Geometry check sheet. Reference: the model listing, model coordinates, mm. Face numbers are marked on the shaded views. A direction names the side the tool comes from. Round coordinates to 2 decimals unless told otherwise and drop trailing zeros. Loops run counter-clockwise (first coordinate to the right, second up) from the corner with the lowest first, then second, coordinate; pieces in that order, holes last. Notation, with made-up numbers: (-26.75, -25.75) -> (-0.75, -25.75) arc R33 cw to (-0.75, 6.25) -> close; hole circle Ø4 at (41.25, 62). An arc over 180 degrees is marked (long way). Use one line per item in the form item = value.
from build123d import *

# Parameters (mm, degrees)
SKETCH1_R           = 95.492297116
BOSS_EXTRUDE1_DEPTH = 100
SKETCH3_3_R         = 32.5
TUBE_DEPTH          = 275
SKETCH5_R           = 82.5
TOP_HUB_DEPTH       = 60
BLADES_DEPTH        = 160
FILLET3_R           = 1.5
FILLET5_R           = 6
FILLET6_R           = 6


with BuildPart() as part:
    # Sketch1 → Boss-Extrude1 (new body)
    with BuildSketch(Plane(origin=(0, 0, 0), x_dir=(1, 0, 0), z_dir=(0, 1, 0))):
        with Locations(Location((0, 0, 0), (0, 0, 270))):
            Circle(SKETCH1_R)
    extrude(amount=BOSS_EXTRUDE1_DEPTH)

    # Loft2: read off the stored shape, not the designer's step
    # Loft2: loft between two sections, ruled curve by curve
    loft2_from = [
        Edge.make_bspline([(30.430707277, 125, -11.411487835), (53.253682947, 125, 49.44992672), (-7.607731608, 125, 72.272902389), (-30.430707277, 125, 11.411487835), (-53.253682947, 125, -49.44992672), (7.607731608, 125, -72.272902389), (30.430707277, 125, -11.411487835)], [0, 0, 0, 0, 0.5, 0.5, 0.5, 1, 1, 1, 1], 3, [1, 0.333333333, 0.333333333, 1, 0.333333333, 0.333333333, 1]),
    ]
    loft2_to = [
        Edge.make_bspline([(87.277179809, 100, 38.748841183), (9.779497444, 100, 213.303200802), (-164.774862175, 100, 135.805518436), (-87.277179809, 100, -38.748841183), (-9.779497444, 100, -213.303200802), (164.774862175, 100, -135.805518436), (87.277179809, 100, 38.748841183)], [0, 0, 0, 0, 0.5, 0.5, 0.5, 1, 1, 1, 1], 3, [1, 0.333333333, 0.333333333, 1, 0.333333333, 0.333333333, 1]),
    ]
    loft2 = Solid(Shell([*[Face.make_surface_from_curves(loft2_from[k], loft2_to[k]) for k in range(1)], Face(Wire(loft2_from)), Face(Wire(loft2_to))]))
    add(loft2)

    # Sketch3<3> → tube (add)
    with BuildSketch(Plane(origin=(0, 125, 0), x_dir=(1, 0, 0), z_dir=(0, 1, 0))):
        with Locations(Location((0, 0, 0), (0, 0, 20.556))):
            Circle(SKETCH3_3_R)
    extrude(amount=TUBE_DEPTH)

    # Sketch5 → top_hub (add)
    with BuildSketch(Plane(origin=(0, 400, 0), x_dir=(1, 0, 0), z_dir=(0, 1, 0))):
        with Locations(Location((0, 0, 0), (0, 0, 270))):
            Circle(SKETCH5_R)
    extrude(amount=TOP_HUB_DEPTH)

    # Sketch8 → Blades (add)
    with BuildSketch(Plane(origin=(0, 460, 0), x_dir=(1, 0, 0), z_dir=(0, 1, 0))):
        with BuildLine():
            ThreePointArc((123.296710019, -36.922200146), (95.784801634, -26.321129354), (82.5, 0))
            ThreePointArc((82.5, 0), (91.565639785, 30.041990229), (119.218910164, 44.874509873))
            Line((119.218910164, 44.874509873), (119.616744296, 40.894343042))
            ThreePointArc((119.616744296, 40.894343042), (94.661353954, 27.508898485), (86.480166831, 0.397834132))
            ThreePointArc((86.480166831, 0.397834132), (98.468890257, -23.355380163), (123.296710019, -32.922200146))
            Line((123.296710019, -32.922200146), (123.296710019, -36.922200146))
        make_face()
        with BuildLine():
            ThreePointArc((-119.218910164, 44.874509873), (-91.565639785, 30.041990229), (-82.5, 0))
            ThreePointArc((-82.5, 0), (-95.784801634, -26.321129354), (-123.296710019, -36.922200146))
            Line((-123.296710019, -36.922200146), (-123.296710019, -32.922200146))
            ThreePointArc((-123.296710019, -32.922200146), (-98.468890257, -23.355380163), (-86.480166831, 0.397834132))
            ThreePointArc((-86.480166831, 0.397834132), (-94.661353954, 27.508898485), (-119.616744296, 40.894343042))
            Line((-119.616744296, 40.894343042), (-119.218910164, 44.874509873))
        make_face()
        with BuildLine():
            ThreePointArc((38.088025782, 119.593401567), (25.871262622, 94.036384856), (0, 82.5))
            ThreePointArc((0, 82.5), (-29.727635854, 92.548615238), (-43.642804778, 120.674672115))
            Line((-43.642804778, 120.674672115), (-39.651708344, 120.941410294))
            ThreePointArc((-39.651708344, 120.941410294), (-27.094116876, 95.559358966), (-0.266738179, 86.491096434))
            ThreePointArc((-0.266738179, 86.491096434), (23.080498822, 96.901980328), (34.105382649, 119.965629555))
            Line((34.105382649, 119.965629555), (38.088025782, 119.593401567))
        make_face()
        with BuildLine():
            ThreePointArc((-43.642804778, -120.674672115), (-29.727635854, -92.548615238), (0, -82.5))
            ThreePointArc((0, -82.5), (25.871262622, -94.036384856), (38.088025782, -119.593401567))
            Line((38.088025782, -119.593401567), (34.105382649, -119.965629555))
            ThreePointArc((34.105382649, -119.965629555), (23.080498822, -96.901980328), (-0.266738179, -86.491096434))
            ThreePointArc((-0.266738179, -86.491096434), (-27.094116876, -95.559358966), (-39.651708344, -120.941410294))
            Line((-39.651708344, -120.941410294), (-43.642804778, -120.674672115))
        make_face()
    extrude(amount=-BLADES_DEPTH)

    # Fillet3
    fillet3_edges = [part.edges().sort_by_distance(p)[0] for p in [
        (123.296710019, 380, 36.922200146),
        (119.218910164, 380, -44.874509873),
        (119.616744296, 380, -40.894343042),
        (123.296710019, 380, 32.922200146),
        (-119.218910164, 380, -44.874509873),
        (-123.296710019, 380, 36.922200146),
        (-123.296710019, 380, 32.922200146),
        (-119.616744296, 380, -40.894343042),
        (38.088025782, 380, -119.593401567),
        (-43.642804778, 380, -120.674672115),
        (-39.651708344, 380, -120.941410294),
        (34.105382649, 380, -119.965629555),
        (-43.642804778, 380, 120.674672115),
        (38.088025782, 380, 119.593401567),
        (34.105382649, 380, 119.965629555),
        (-39.651708344, 380, 120.941410294),
    ]]
    fillet(fillet3_edges, radius=FILLET3_R)

    # Fillet5
    fillet5_edges = [part.edges().sort_by_distance(p)[0] for p in [
        (52.050758656, 100, 80.059336319),
        (-30.430707277, 125, 11.411487835),
    ]]
    fillet(fillet5_edges, radius=FILLET5_R)

    # Fillet6
    fillet6_edges = [part.edges().sort_by_distance(p)[0] for p in [
        (-30.430707277, 400, 11.411487835),
    ]]
    fillet(fillet6_edges, radius=FILLET6_R)


solid = part.part
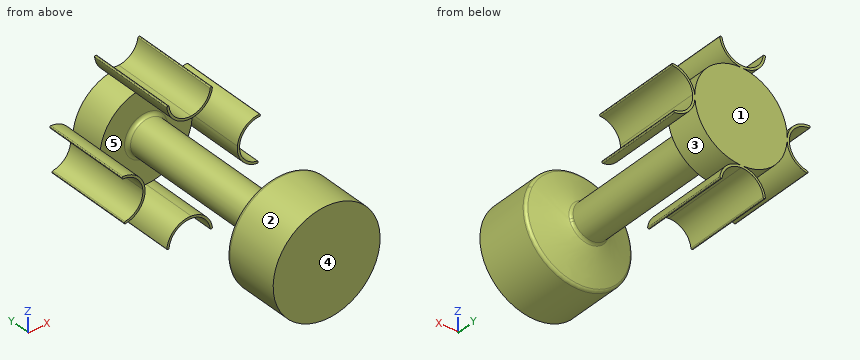
1. Mould release check, pull along Z, two halves, no side actions. Record for the marked faces 1, 2 and 3: released by +Z, released by -Z, zero draft, split by the parting line, or undercut.
Return value:
face_1 = zero draft
face_2 = split by the parting line
face_3 = undercut
2. Gauge pin test, flat ends, axial feed: pin 1 (6 mm diameter, centred on x = -93.5, y = 399.5, fed in from -Z); pin 2 (12 mm diameter, centred on y = 404.5, z = 79, fed in from -X) (3 decimals); pin 3 (2 mm diameter, centred on y = 404.5, z = 70, fed in from +X); pin 4 (5 mm diameter, centred on x = 53.5, z = 9.5, fed in from -Y). Record the tip position at first contact, or that the pin passes through.
Return value:
pin_1 = -35.11
pin_2 = -38.435
pin_3 = 45.22
pin_4 = 0
3. Section check A-A (z = 102.5). Record the boundary of the cut face in (x, y).
Return value:
outline = (-38, 300) -> (-33.26, 300) -> (-33.26, 460) -> (-38, 460) -> close; (27.79, 300) -> (32.53, 300) -> (32.53, 460) -> (27.79, 460) -> close
4. Tool access check on the marked faces 4 and 5. Record the directions out of +Z, -Z, +X, -X, +Y, -Y that give a thin tool (end or side, any length) a straight path to the whole face; none if there is none.
Return value:
face_4 = +Z, -Z, +X, -X, -Y
face_5 = none
5. Section check C-C (y = 243). Record the boundary of the cut face in (x, z), then the cut area to 3 significant figures.
Return value:
outline = circle Ø65 at (0, 0)
area = 3,320 mm2
6. Section check B-B (x = -13). Count the separate pieces of the cut face and the enclosed holes in it, then the cut area to 3 significant figures.
Return value:
separate_pieces = 3
enclosed_holes = 0
area = 49,400 mm2
7. Material ranges on line 1 along Z through (x, y) = (11, 405); line 2 along X through (y, z) = (417.5, -21); line 3 along X through (y, z) = (391, 14.5), recorded low to high.
Return value:
line_1 = -89.05 to -84.78, -81.76 to 81.76, 84.78 to 89.05
line_2 = -90.39 to -85.95, -79.78 to 79.78, 85.95 to 90.39
line_3 = -91.3 to -86.75, -29.09 to 29.09, 86.75 to 91.3
